For this review, take the finished solid that the model builds, in its own axes (mm). Coordinates: 2 decimals unless noted, no trailing zeros. Loops run counter-clockwise (first coordinate to the right, second up) from the corner with the lowest first, then second, coordinate; pieces in that order, holes last. Notation, with made-up numbers: (-23, 59) - (33, 59) arc R30 cw to (33, 95) - close; hole circle Ø5 at (-13.75, -23). An arc over 180 degrees is marked (long way). Use one line per item in the form item = value. Start each with the question number.
1. Add section C-C on y = 0. Count the separate pieces of the cut face and the enclosed holes in it, and give its area (3 significant figures).
2. Add section B-B on z = 37. Give the boundary of the cut face in (x, y).
3. Add section D-D on z = 22.5. Give the boundary of the cut face in (x, y).
4. To check wall thickness, follow probe 1 along Z at (x, y) = (0, -4.6); probe 2 along X at (y, z) = (-2, 26.5); probe 3 along Y at (x, z) = (4.45, 5). State the ranges of each line that lie inside material, in increasing order.
5. Add section A-A on x = 0. Give the boundary of the cut face in (y, z).
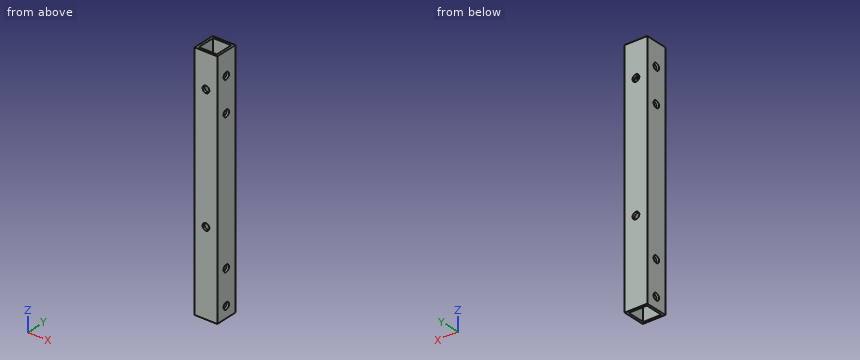
```python
from build123d import *

# Parameters (mm, degrees)
SKETCH_1_W          = 10
SKETCH_1_H          = 10
SKETCH_1_W_2        = 8
SKETCH_1_H_2        = 8
EXTRUDE_1_DEPTH     = 107
SKETCH_2_R          = 1.5
CUT_EXTRUDE_1_DEPTH = 11
SKETCH_3_R          = 1.5
CUT_EXTRUDE_2_DEPTH = 10


with BuildPart() as part:
    # 草图1 → 拉伸-薄壁1 (new body)
    with BuildSketch(Plane.XY):
        Rectangle(SKETCH_1_W, SKETCH_1_H)
        Rectangle(SKETCH_1_W_2, SKETCH_1_H_2, mode=Mode.SUBTRACT)
    extrude(amount=EXTRUDE_1_DEPTH)

    # 草图2 → 切除-拉伸1 (cut, through all)
    with BuildSketch(Plane(origin=(5, 0, 0), x_dir=(0, 0, -1), z_dir=(1, 0, 0))):
        with Locations((-5, 0)):
            Circle(SKETCH_2_R)
        with Locations((-20, 0)):
            Circle(SKETCH_2_R)
        with Locations((-97, 0)):
            Circle(SKETCH_2_R)
        with Locations((-82, 0)):
            Circle(SKETCH_2_R)
    extrude(amount=-CUT_EXTRUDE_1_DEPTH, mode=Mode.SUBTRACT)

    # 草图3 → 切除-拉伸2 (cut)
    with BuildSketch(Plane.XZ.offset(5)):
        with Locations((0, 92)):
            Circle(SKETCH_3_R)
        with Locations((0, 37)):
            Circle(SKETCH_3_R)
    extrude(amount=-CUT_EXTRUDE_2_DEPTH, mode=Mode.SUBTRACT)


solid = part.part
```
Conclusion:
q1.separate_pieces = 10
q1.enclosed_holes = 0
q1.area = 190 mm^2
q2.outline = (-5, -5) - (-1.5, -5) - (-1.5, -4) - (-4, -4) - (-4, 4) - (-1.5, 4) - (-1.5, 5) - (-5, 5) - close; (1.5, -5) - (5, -5) - (5, 5) - (1.5, 5) - (1.5, 4) - (4, 4) - (4, -4) - (1.5, -4) - close
q3.outline = (-5, -5) - (5, -5) - (5, 5) - (-5, 5) - close; hole (-4, -4) - (4, -4) - (4, 4) - (-4, 4) - close
q4.probe_1 = 0 to 35.5, 38.5 to 90.5, 93.5 to 107
q4.probe_2 = -5 to -4, 4 to 5
q4.probe_3 = -5 to -1.5, 1.5 to 5
q5.outline = (-5, 0) - (-4, 0) - (-4, 35.5) - (-5, 35.5) - close; (-5, 38.5) - (-4, 38.5) - (-4, 90.5) - (-5, 90.5) - close; (-5, 93.5) - (-4, 93.5) - (-4, 107) - (-5, 107) - close; (4, 0) - (5, 0) - (5, 35.5) - (4, 35.5) - close; (4, 38.5) - (5, 38.5) - (5, 90.5) - (4, 90.5) - close; (4, 93.5) - (5, 93.5) - (5, 107) - (4, 107) - close
